CAD build for the part. Positions are in the model's coordinates, mm. A direction names the side the tool comes from. Coordinates: 2 decimals unless noted, no trailing zeros. Write each loop counter-clockwise with the first axis right and the second up, starting at its lowest first coordinate (ties: lowest second). Pieces come first, ordered by that corner, then holes. Notation, with made-up numbers: (-14.75, -14.5) -> (6.25, -14.5) arc R16 ccw to (6.25, 11.5) -> close; hole circle Ø5 at (4.25, 89.5). An arc over 180 degrees is marked (long way). Answer as CSV lines item,"result". Start each with the question number.
```python
from build123d import *

# Parameters (mm, degrees)
PAD_DEPTH = 75


with BuildPart() as part:
    # Sketch → Pad (new body)
    with BuildSketch(Plane.XY):
        with BuildLine():
            ThreePointArc((-29.848016, -3.015947), (29.920505, -2.182515), (-29.094406, 7.315431))
            ThreePointArc((-29.094406, 7.315431), (-29.072912, 3.034578), (-26.991574, -0.706304))
            Line((-26.991574, -0.706304), (-12.739759, -15.728805))
            ThreePointArc((-12.739759, -15.728805), (-11.4789, -15.911046), (-11.008743, -14.727014))
            Line((-11.008743, -14.727014), (-18.604437, 10.709188))
            ThreePointArc((-18.160969, 13.282665), (-18.684551, 12.047942), (-18.604437, 10.709188))
            ThreePointArc((-20.499669, -9.27435), (22.380035, -2.320351), (-18.160969, 13.282665))
            ThreePointArc((-20.499669, -9.27435), (-21.232479, -7.959372), (-22.173804, -6.784601))
            Line((-22.173804, -6.784601), (-26.991574, -1.706304))
            ThreePointArc((-26.991574, -1.706304), (-28.888073, -1.339771), (-29.848016, -3.015947))
        make_face()
    extrude(amount=PAD_DEPTH)


solid = part.part
```
1. Cut at C-C (x = 19). Give the cut face in (y, z).
2. Tool access for faces 1 (the face through (-14.753, -2.187, 36.975)), 2 (the face through (-14, -6, 0)): list every direction of +Z, -Z, +X, -X, +Y, -Y with a clear straight run to the whole face (end or side of a thin tool).
3. Cut at A-A (x = 0). Give the cut face in (y, z).
4. Cut at B-B (z = 61). Give the cut face in (x, y).
5. Flat gauge pins, fed straight in: P1, Ø12, axis at x = -21.5, z = 13, coming from the +Y side; P2, Ø1.5, axis at y = 11, z = 67, coming from the +X side; P3, Ø2, axis at x = -20, z = 27, coming from the -Y side. Where does each tip first touch, or does it go through?
6. Mould opens along X. For faces 3 (the face through (-21.22, -7.98, 36.98)), 4 (the face through (29.804, -3.424, 36.975)), 5 (the face through (-29.088, 3.093, 36.975)) say: pulls with the +X half, pulls with the -X half, needs draft (parallel to the pull), parting line crosses it, or undercut.
7. Cut at D-D (y = -25). Give the cut face in (x, z), then the cut area to 3 significant figures.
8. Wall check: line 1 (Y direction, x = 0, z = 45.5); line 2 (X direction, y = -13, z = 5); line 3 (X direction, y = -8, z = 52). Give the ranges that are in metal, low to high.
Geometry check:
1,outline,"(-23.22, 0) -> (-12.05, 0) -> (-12.05, 75) -> (-23.22, 75) -> close; (12.05, 0) -> (23.22, 0) -> (23.22, 75) -> (12.05, 75) -> close"
2,face 1,"+Z, -Z"
2,face 2,"-Z, +X, -X, +Y, -Y"
3,outline,"(-30, 0) -> (-22.5, 0) -> (-22.5, 75) -> (-30, 75) -> close; (22.5, 0) -> (30, 0) -> (30, 75) -> (22.5, 75) -> close"
4,outline,"(-29.85, -3.02) arc R30 ccw (long way) to (-29.09, 7.32) arc R8.61 ccw to (-26.99, -0.71) -> (-12.74, -15.73) arc R1.03 ccw to (-11.01, -14.73) -> (-18.6, 10.71) arc R2.94 cw to (-18.16, 13.28) arc R22.5 cw (long way) to (-20.5, -9.27) arc R9.02 ccw to (-22.17, -6.78) -> (-26.99, -1.71) arc R1.66 ccw to start"
5,P1,"y = 25.69"
5,P2,"x = 28.19"
5,P3,"y = -23.22"
6,face 3,"undercut"
6,face 4,"parting line crosses it"
6,face 5,"pulls with the -X half"
7,outline,"(-16.58, 0) -> (16.58, 0) -> (16.58, 75) -> (-16.58, 75) -> close"
7,area,"2,490 mm²"
8,line 1,"-30 to -22.5, 22.5 to 30"
8,line 2,"-27.04 to -18.36, -15.33 to -11.52, 18.36 to 27.04"
8,line 3,"-28.91 to -21.21, -20.07 to -13.02, 21.03 to 28.91"
